Input: part model. Units: mm. Frame: model coordinates. Face numbers are marked on the shaded views. A direction names the side the tool comes from. Give positions to 0.01 mm unless a question says otherwise; leave off trailing zeros. Order: outer loops, then holes, each group sorted by start corner. A loop starts at its lowest first (then second) coordinate and runs counter-clockwise, first axis right, second up. Notation, with made-up numbers: (-35.75, 22.5) - (12.25, 22.5) arc R30 cw to (12.25, 47.5) - close; hole circle Ø5 at (-19.75, 84). An arc over 180 degrees is marked (long way). Answer in a Markdown table with one row per item. Add a question column.
1. Contact query for flat-ended pins moving along their axis: pin 1 (5 mm diameter, centred on x = -6.5, y = 9, fed in from +Z); pin 2 (5 mm diameter, centred on x = 0, z = 4.5, fed in from +Y); pin 3 (12 mm diameter, centred on x = -8.5, y = 8, fed in from -Z). Output: stop coordinate, or through.
2. Ray query, line 1 (Z direction, x = 0, y = 6); line 2 (X direction, y = 4.75, z = 1.5); line 3 (X direction, y = 4, z = 4). Return the intervals inside material, ascending. Write a range as [from, to].
3. Access query for the marked faces 1 and 2. Directions: +Z, -Z, +X, -X, +Y, -Y. A direction counts if a zero-diameter tool reaches every point of the face in a straight line with its end or side. Return the directions, or none.
4. Section query C-C on z = 0. Return loops of the section in (x, y).
5. Mould query, pull axis X, two halves, no side actions, for the marked faces 3, 4 and 5. Classes: released by +X, released by -X, zero draft, split by the parting line, or undercut.
6. Section query D-D on y = 15.5. Return loops of the section in (x, z), and give its area (3 significant figures).
7. Section query B-B on x = 0. Return loops of the section in (y, z).
8. Section query A-A on y = 3.75. Return loops of the section in (x, z).
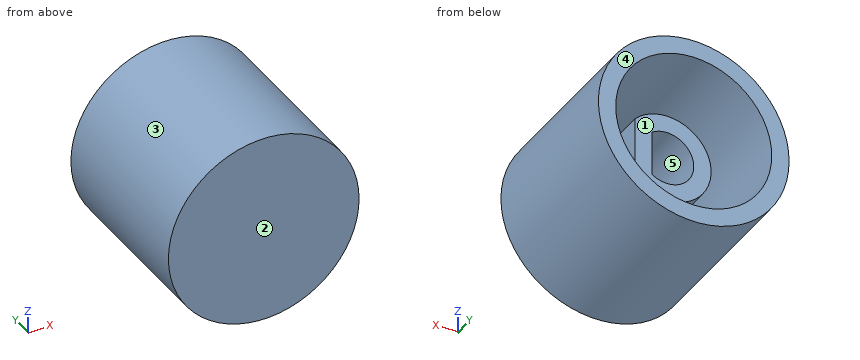
Autodesk Fusion 360 part; units mm, degrees
sketch "Outer" plane through (0, 0, 0) normal (0, 1, 0) x (1, 0, 0)
  circle A0 centre (0, 0) radius 11
  dimension "d1" = 22
extrude "Outer Extrusion" add sketch "Outer" along normal blind 20
sketch "Inner" plane through (0, 20, 0) normal (0, 1, 0) x (-1, 0, 0)
  circle A0 centre (0, 0) radius 11
  circle A1 centre (0, 0) radius 9
  dimension "d4" = 18
extrude "Inner Extrusion" cut sketch "Inner" against normal blind 18 contours A1
sketch "Shaft" plane through (0, 2, 0) normal (0, 1, 0) x (-1, 0, 0)
  circle A0 centre (0, 0) radius 9
  line L0 (-1.7, 2.5923) -> (-1.7, -2.5923)
  arc A1 (-1.7, -2.5923) -> (-1.7, 2.5923) centre (0, 0) ccw
  arc A2 (-3.7, -3.51) -> (-3.7, 3.51) centre (0, 0) ccw
  line L1 (-3.7, 3.51) -> (-3.7, -3.51)
  dimension "d7" = 6.2
  dimension "d8" = 1.7
  dimension "d9" = 2
extrude "Shaft Extrusion" add sketch "Shaft" along normal blind 12.5 contours A2 L1
equation "d5 = -( 20 mm - 2 mm )"
equation "d7 = 5.8 mm + 0.2 mm + 0.2 mm"
equation "d8 = ( 4.5 mm - 3 mm ) + 0.2 mm"
equation "d10 = 20 mm - 2 mm - 5.5 mm"
equation "d14 = 20 mm - 2 mm - 5.5 mm"
Answer:
| question | item | result |
|---|---|---|
| 1 | pin 1 | stops at z = 10.25 |
| 1 | pin 2 | stops at y = 14.5 |
| 1 | pin 3 | stops at z = -10.71 |
| 2 | line 1 | z = [-11, -9], [-5.1, -3.1], [3.1, 5.1], [9, 11] |
| 2 | line 2 | x = [-10.9, -8.87], [-4.87, -2.71], [1.7, 3.7], [8.87, 10.9] |
| 2 | line 3 | x = [-10.25, -8.06], [-3.16, 3.16], [8.06, 10.25] |
| 3 | face 1 | +Y |
| 3 | face 2 | +Z, -Z, +X, -X, -Y |
| 4 | outline | (-11, 0) - (11, 0) - (11, 20) - (9, 20) - (9, 2) - (3.7, 2) - (3.7, 14.5) - (1.7, 14.5) - (1.7, 2) - (-3.1, 2) - (-3.1, 14.5) - (-5.1, 14.5) - (-5.1, 2) - (-9, 2) - (-9, 20) - (-11, 20) - close |
| 5 | face 3 | split by the parting line |
| 5 | face 4 | zero draft |
| 5 | face 5 | undercut |
| 6 | outline | circle Ø22 at (0, 0); hole circle Ø18 at (0, 0) |
| 6 | area | 126 mm² |
| 7 | outline | (0, -11) - (20, -11) - (20, -9) - (2, -9) - (2, -5.1) - (14.5, -5.1) - (14.5, -3.1) - (2, -3.1) - (2, 3.1) - (14.5, 3.1) - (14.5, 5.1) - (2, 5.1) - (2, 9) - (20, 9) - (20, 11) - (0, 11) - close |
| 8 | outline | circle Ø22 at (0, 0); (3.7, -3.51) - (3.7, 3.51) arc R5.1 ccw (long way) to start; hole circle Ø18 at (0, 0); hole (1.7, -2.59) - (1.7, 2.59) arc R3.1 ccw (long way) to start |
